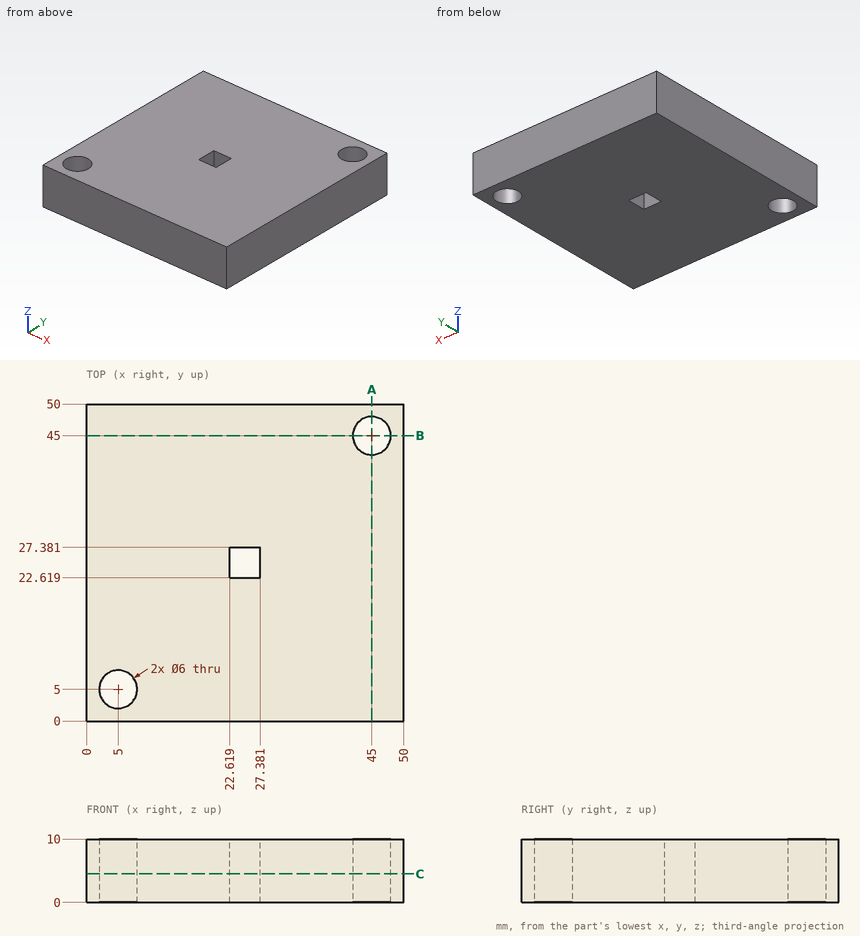
Geometry check sheet. Reference: drawing and pictorial views, mm from the part's lowest x, y, z. Give positions to 0.01 mm unless a question says otherwise; leave off trailing zeros. Write each loop counter-clockwise with the first axis right and the second up, starting at its lowest first coordinate (ties: lowest second). Pieces come first, ordered by that corner, then holes.
Item 1: Cross-section at C-C (z = 4.5). Enter the section's corners in (x, y).
Item 2: Cross-section at A-A (x = 45). Enter the section's corners in (y, z).
Item 3: Gauge pin test, flat end, axial feed: pin 1 (3.5 mm diameter, centred on x = 5, y = 5, fed in from +Z). Record the tip position at first contact, or that the pin passes through.
Item 4: Scan lines: L1, parallel to Y at x = 25, z = 2.75; L2, parallel to Y at x = 45, z = 7. Record each from-to range of solid material in increasing order.
Report:
1. outline: (0, 0) - (50, 0) - (50, 50) - (0, 50) - close; hole circle Ø6 at (5, 5); hole (22.62, 22.62) - (27.38, 22.62) - (27.38, 27.38) - (22.62, 27.38) - close; hole circle Ø6 at (45, 45)
2. outline: (0, 0) - (42, 0) - (42, 10) - (0, 10) - close; (48, 0) - (50, 0) - (50, 10) - (48, 10) - close
3. pin 1: passes through
4. L1: y = 0 to 22.62, 27.38 to 50
4. L2: y = 0 to 42, 48 to 50
